Build history of the part. All positions in model axes, mm. Face numbers are marked on the shaded views. A direction names the side the tool comes from. Coordinates: 2 decimals unless noted, no trailing zeros. Order: outer loops, then holes, each group sorted by start corner. A loop starts at its lowest first (then second) coordinate and runs counter-clockwise, first axis right, second up. Notation, with made-up numbers: M 18,68 L 54,68 A19 ccw 54,81 Z; hole C -31.5,29 d3. An arc over 180 degrees is marked long. Write item = value, one per line. Start each with the question number.
Q1. Drill centre lines: probe 1 along X at (y, z) = (-2.5, 1.75); probe 2 along Y at (x, z) = (32, 0.75); probe 3 along Y at (x, z) = (8, 3.05). Where is each one in solid material? Low to high.
Q2. Band-saw the part on A-A on z = 2.2. Write the cut outline in (x, y), plus the area to 3 significant figures.
Q3. Pin check, flat tips, straight feed: P1, Ø1.6, axis at y = 18.5, z = 2, coming from the +X side; P2, Ø1.6, axis at x = 37, z = 2, coming from the +Y side; P3, Ø1, axis at y = -3, z = 2, coming from the +X side. Stop position of each tip, or through.
Q4. 3-axis set-ups, long thin cutter, end or side, ignore diameter. For the marked faces 1, 2, 3 and 4: which of +Z, -Z, +X, -X, +Y, -Y reach the whole face in a straight line?
Q5. Band-saw the part on B-B on x = 36. Write the cut outline in (y, z).
Q6. Pull direction X, two halves, no side cores. Call the marked faces 5, 6, 7 and 8: released by +X, released by -X, zero draft, split by the parting line, or undercut.
Q7. Band-saw the part on C-C on y = 3. Write the cut outline in (x, z), plus the area to 4 significant figures.
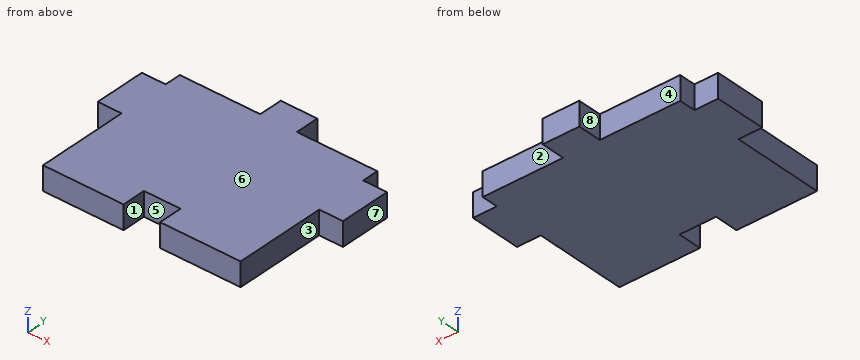
Autodesk Inventor part; units mm, degrees
ref_plane "YZ Plane" through (0, 0, 0) normal (1, 0, 0) x (0, 1, 0)
ref_plane "XZ Plane" through (0, 0, 0) normal (0, 1, 0) x (-1, 0, 0)
ref_plane "XY Plane" through (0, 0, 0) normal (0, 0, 1) x (1, 0, 0)
sketch "Block1" plane through (0, 0, 0) normal (0, 0, 1) x (1, 0, 0)
  circle A0 centre (74.029, 24.2723) radius 1
  line L0 (49.279, 30.4723) -> (71.779, 30.4723)
  line L1 (71.779, 30.4723) -> (71.779, 18.0723)
  line L2 (71.779, 18.0723) -> (49.279, 18.0723)
  line L3 (49.279, 18.0723) -> (49.279, 30.4723)
  line L4 (49.279, 30.4723) -> (44.779, 30.4723)
  line L5 (44.779, 30.4723) -> (44.779, 18.0723)
  line L6 (44.779, 18.0723) -> (49.279, 18.0723)
  line L7 (49.279, 18.0723) -> (49.279, 30.4723)
  line L8 (71.779, 30.4723) -> (76.279, 30.4723)
  line L9 (76.279, 30.4723) -> (76.279, 18.0723)
  line L10 (76.279, 18.0723) -> (71.779, 18.0723)
  line L11 (71.779, 18.0723) -> (71.779, 30.4723)
  line L12 (44.779, 24.2723) -> (76.279, 24.2723) construction
  line L13 (47.029, 30.4723) -> (47.029, 18.0723) construction
  circle A1 centre (47.029, 24.2723) radius 1
  line L14 (74.029, 30.4723) -> (74.029, 18.0723) construction
  point P0 (60.979, 24.0984)
  dimension "d7" = 22.5
  dimension "d8" = 12.4
  dimension "d9" = 4.5
  dimension "d10" = 4.5
  dimension "d11" = 2
  dimension "d12" = 2
sketch "Sketch1" plane through (0, 0, 0) normal (0, 0, 1) x (1, 0, 0)
  line L0 (-92.7646, -8.503) -> (-89.7646, -8.503)
  line L1 (-89.7646, -8.503) -> (-89.7646, -11.753)
  line L2 (-89.7646, -11.753) -> (-92.7646, -11.753)
  line L3 (-92.7646, -11.753) -> (-92.7646, -8.503)
  line L4 (-92.7646, -21.6527) -> (-89.7646, -21.6527)
  line L5 (-89.7646, -21.6527) -> (-89.7646, -21.7527)
  line L6 (-89.7646, -21.7527) -> (-92.7646, -21.7527)
  line L7 (-92.7646, -21.7527) -> (-92.7646, -21.6527)
  line L8 (8.2387, -5.1967) -> (35.2387, -5.1967)
  line L9 (35.2387, -5.1967) -> (35.2387, 16.5533)
  line L10 (35.2387, 16.5533) -> (8.2387, 16.5533)
  line L11 (8.2387, 16.5533) -> (8.2387, -5.1967)
  line L12 (8.2387, 5.6783) -> (35.2387, 5.6783) construction
  line L13 (21.7387, 16.5533) -> (21.7387, -5.1967) construction
  line L14 (19.2387, 16.5533) -> (24.2387, 16.5533)
  line L15 (24.2387, 16.5533) -> (24.2387, 19.8033)
  line L16 (24.2387, 19.8033) -> (19.2387, 19.8033)
  line L17 (19.2387, 19.8033) -> (19.2387, 16.5533)
  line L18 (21.7387, 19.8033) -> (21.7387, 16.5533) construction
  line L19 (8.2387, 14.3033) -> (4.9887, 14.3033)
  line L20 (4.9887, 14.3033) -> (4.9887, 7.3033)
  line L21 (4.9887, 7.3033) -> (8.2387, 7.3033)
  line L22 (8.2387, 7.3033) -> (8.2387, 14.3033)
  line L23 (19.2387, -5.1967) -> (24.2387, -5.1967)
  line L24 (24.2387, -5.1967) -> (24.2387, -1.9467)
  line L25 (24.2387, -1.9467) -> (19.2387, -1.9467)
  line L26 (19.2387, -1.9467) -> (19.2387, -5.1967)
  line L27 (21.7387, -1.9467) -> (21.7387, -5.1967) construction
  line L28 (35.2387, 14.3033) -> (38.4887, 14.3033)
  line L29 (38.4887, 14.3033) -> (38.4887, 7.3033)
  line L30 (38.4887, 7.3033) -> (35.2387, 7.3033)
  line L31 (35.2387, 7.3033) -> (35.2387, 14.3033)
  point P0 (0, 0)
  dimension "d0" = 3
  dimension "mat" = 3.25
  dimension "d2" = 3
  dimension "d3" = 0.1
  dimension "d58" = 27
  dimension "d59" = 21.75
  dimension "d60" = 5
  dimension "d61" = 3.25
  dimension "d64" = 3.25
  dimension "d65" = 7
  dimension "d66" = 5
  dimension "d67" = 3.25
  dimension "d70" = 2.25
  dimension "d75" = 27
extrude "Extrusion5" add sketch "Sketch1" along normal blind 3.25 contours L11 L10 L9 L8 L24 L25 L26 | L26 L25 L24 L8 | L17 L16 L15 L10
extrude "Extrusion6" cut sketch "Sketch1" along normal blind 3.25 contours L26 L25 L24 L8
extrude "Extrusion7" add sketch "Sketch1" along normal blind 3.25 contours L21 L20 L19 L11
extrude "Extrusion8" add sketch "Sketch1" along normal blind 3.25 contours L9 L28 L29 L30
equation "\"d61\" = mat"
equation "\"d64\" = mat"
equation "\"d67\" = mat"
equation "\"d62\" = mat"
equation "\"d68\" = mat"
equation "\"d71\" = mat"
equation "\"d73\" = mat"
properties part number "arm-servo"
Recorded:
q1.probe_1 = 8.24 to 19.24, 24.24 to 35.24
q1.probe_2 = -5.2 to 16.55
q1.probe_3 = 7.3 to 14.3
q2.outline = M 4.99,7.3 L 8.24,7.3 L 8.24,-5.2 L 19.24,-5.2 L 19.24,-1.95 L 24.24,-1.95 L 24.24,-5.2 L 35.24,-5.2 L 35.24,7.3 L 38.49,7.3 L 38.49,14.3 L 35.24,14.3 L 35.24,16.55 L 24.24,16.55 L 24.24,19.8 L 19.24,19.8 L 19.24,16.55 L 8.24,16.55 L 8.24,14.3 L 4.99,14.3 Z
q2.area = 633 mm2
q3.P1 = 24.24
q3.P2 = 14.3
q3.P3 = 35.24
q4.face_1 = +Z, -Z, -Y
q4.face_2 = +Z, -Z, +X, +Y
q4.face_3 = +Z, -Z, +X, -Y
q4.face_4 = +Z, -Z, -X, +Y
q5.outline = M 7.3,0 L 14.3,0 L 14.3,3.25 L 7.3,3.25 Z
q6.face_5 = undercut
q6.face_6 = zero draft
q6.face_7 = released by +X
q6.face_8 = released by -X
q7.outline = M 8.24,0 L 35.24,0 L 35.24,3.25 L 8.24,3.25 Z
q7.area = 87.75 mm2
